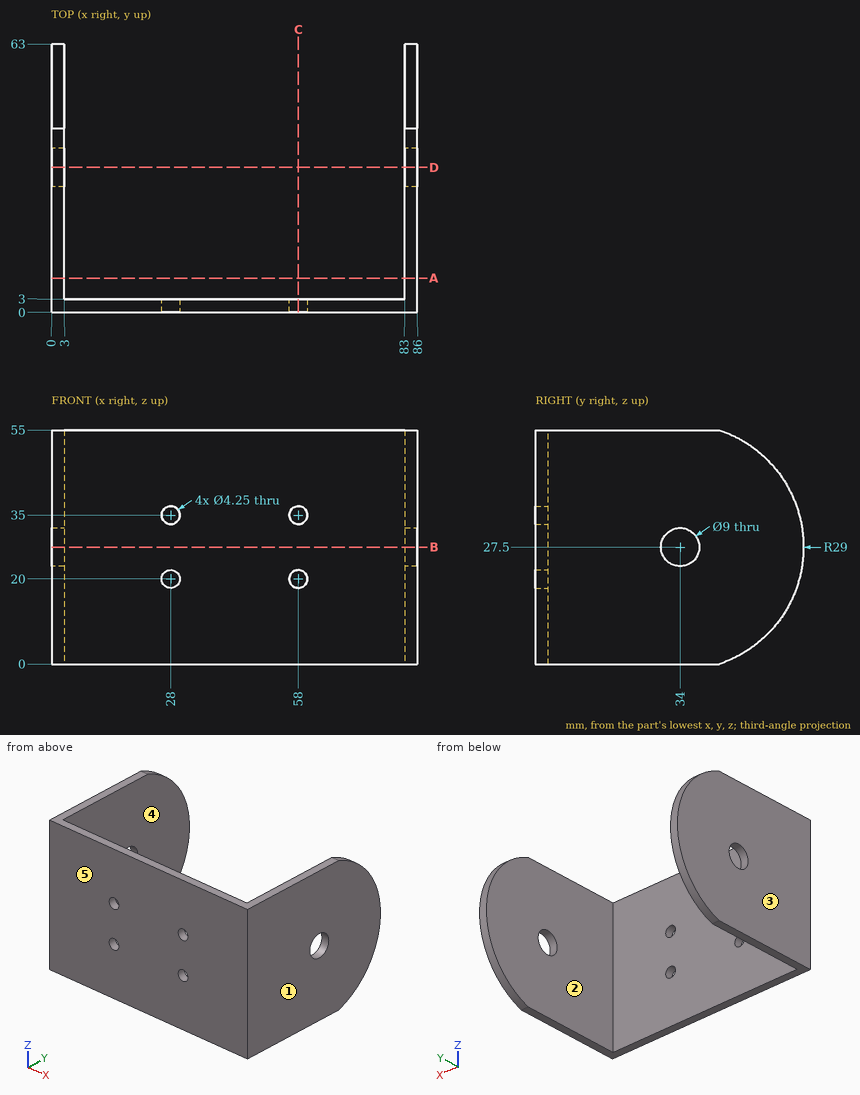
Geometry: see drawing. Coordinates: mm, zero at the bounding-box minimum. A direction names the side the tool comes from. Give positions to 0.01 mm unless a question says otherwise; leave off trailing zeros. Write each loop counter-clockwise with the first axis right and the second up, starting at its lowest first coordinate (ties: lowest second). Pieces come first, ordered by that corner, then holes. Notation, with made-up numbers: M -11.75,4.5 L 14.25,4.5 A18 ccw 14.25,38.5 Z; hole C 78.5,34.5 d2. An arc over 180 degrees is marked long. Answer in a Markdown table with one row per item. Add a question column.
(1) Section B-B on z = 27.5. Return loops of the section in (x, y).
(2) First-contact query: pin 1 (1.5 mm diameter, centred on x = 59, z = 24.5, fed in from +Y); pin 2 (1 mm diameter, centred on x = 68, z = 47.5, fed in from -Y). Flat tips, straight axial feed; report the tip coordinate or a pass-through.
(3) Section D-D on y = 34. Return loops of the section in (x, z), and give its area (3 significant figures).
(4) Section A-A on y = 8. Return loops of the section in (x, z), and give its area (3 significant figures).
(5) Mould query, pull axis X, two halves, no side actions, for the marked faces 3, 4 and 5. Classes: +X half, -X half, draft (parallel to the pull), parting line (faces both ways), or undercut.
(6) Reachability of the marked faces 1 and 2 from +Z, -Z, +X, -X, +Y, -Y: full face, straight path, thin tool, end or side. Return the list, or none.
(7) Section C-C on x = 58. Return loops of the section in (y, z) (3 decimals), and give its area (4 significant figures).
(8) Ray query, line 1 (X direction, y = 1.6, z = 35) (3 decimals); line 2 (X direction, y = 15, z = 31.5); line 3 (Y direction, x = 55, z = 8.5). Return the intervals inside material, ascending.
Result set:
| question | item | result |
|---|---|---|
| 1 | outline | M 0,0 L 86,0 L 86,29.5 L 83,29.5 L 83,3 L 3,3 L 3,29.5 L 0,29.5 Z; M 0,38.5 L 3,38.5 L 3,63 L 0,63 Z; M 83,38.5 L 86,38.5 L 86,63 L 83,63 Z |
| 2 | pin 1 | stops at y = 3 |
| 2 | pin 2 | stops at y = 0 |
| 3 | outline | M 0,0 L 3,0 L 3,23 L 0,23 Z; M 0,32 L 3,32 L 3,55 L 0,55 Z; M 83,0 L 86,0 L 86,23 L 83,23 Z; M 83,32 L 86,32 L 86,55 L 83,55 Z |
| 3 | area | 276 mm^2 |
| 4 | outline | M 0,0 L 3,0 L 3,55 L 0,55 Z; M 83,0 L 86,0 L 86,55 L 83,55 Z |
| 4 | area | 330 mm^2 |
| 5 | face 3 | -X half |
| 5 | face 4 | undercut |
| 5 | face 5 | draft |
| 6 | face 1 | +Z, -Z, +X, +Y, -Y |
| 6 | face 2 | +Z, -Z, +Y |
| 7 | outline | M 0,0 L 3,0 L 3,17.875 L 0,17.875 Z; M 0,22.125 L 3,22.125 L 3,32.875 L 0,32.875 Z; M 0,37.125 L 3,37.125 L 3,55 L 0,55 Z |
| 7 | area | 139.5 mm^2 |
| 8 | line 1 | x = 0 to 25.875, 30.125 to 55.875, 60.125 to 86 |
| 8 | line 2 | x = 0 to 3, 83 to 86 |
| 8 | line 3 | y = 0 to 3 |
